```python
from build123d import *

# Parameters (mm, degrees)
F0_W        = 50
F0_H        = 50
F1_DEPTH    = 80
F2_T1_DEPTH = 27.2793198937
F2_T3_DEPTH = 202.8653193294
F2_T5_DEPTH = 172.8653193294
F2_T7_DEPTH = 172.8653193294
F3_SIZE     = 25
F4_SIZE     = 10
F5_SIZE     = 20


# Not quite as in the source:
# - a fillet or chamfer that OpenCascade refuses, or shapes differently, is made with other operations: its cross-section is extruded or revolved along the edge and cut away or added


with BuildPart() as f1:
    # F0 (on Top) → F1 (new body)
    with BuildSketch(Plane.XY):
        Rectangle(F0_W, F0_H)
    extrude(amount=F1_DEPTH)

    # F2: chamfer of 20 x 23.8350718519 on 3 edges, made by hand

    # F2_s2 → F2_t1 (cut)
    with BuildSketch(Plane(origin=(23.3481641649, -33.1608518108, 27.825258524), x_dir=(0.8176584321, 0.5757036463, 0), z_dir=(0.4747146788, -0.6742261621, 0.565742924))):
        Polygon((-13.4400778356, 34.368541497), (17.5629425707, 39.0194717243), (-1.9260049086, 63.2741944877), align=None)
    extrude(amount=F2_T1_DEPTH, mode=Mode.SUBTRACT)

    # F2_s4 → F2_t3 (cut)
    with BuildSketch(Plane.XY.offset(-61.4326596647)):
        Polygon((1.1649281481, -25), (25, -5), (25, -25), align=None)
    extrude(amount=F2_T3_DEPTH, mode=Mode.SUBTRACT)

    # F2_s6 → F2_t5 (cut)
    with BuildSketch(Plane.XZ.offset(-86.4326596647)):
        Polygon((25, 60), (1.1649281481, 80), (25, 80), align=None)
    extrude(amount=F2_T5_DEPTH, mode=Mode.SUBTRACT)

    # F2_s8 → F2_t7 (cut)
    with BuildSketch(Plane.YZ.offset(-86.4326596647)):
        Polygon((-25, 56.1649281481), (-5, 80), (-25, 80), align=None)
    extrude(amount=F2_T7_DEPTH, mode=Mode.SUBTRACT)

    # F3
    f3_edges = [f1.edges().sort_by_distance(p)[0] for p in [
        (-25, 25, 40),
    ]]
    chamfer(f3_edges, length=F3_SIZE)

    # F4
    f4_edges = [f1.edges().sort_by_distance(p)[0] for p in [
        (-12.5, 12.5, 80),
    ]]
    chamfer(f4_edges, length=F4_SIZE)

    # F5
    f5_edges = [f1.edges().sort_by_distance(p)[0] for p in [
        (12.5, 25, 0),
        (-11.917536, -25, 0),
    ]]
    chamfer(f5_edges, length=F5_SIZE)


solid = f1.part
```
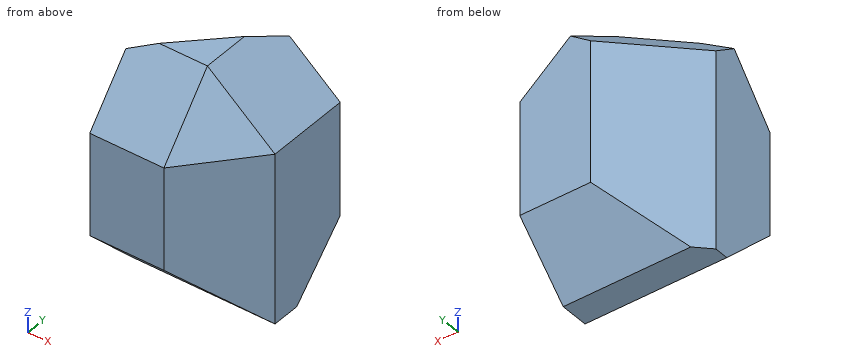
Source: CAD feature listing. Evaluate the final solid. Frame: model axes, mm. Round coordinates to 2 decimals unless told otherwise and drop trailing zeros. Loops run counter-clockwise (first coordinate to the right, second up) from the corner with the lowest first, then second, coordinate; pieces in that order, holes last.
(1) Section query A-A (x = 12.5). Output: boundary loops of the cut face in (y, z).
From the geometry:
outline: (-15.49, 10.49) - (-5, 0) - (5, 0) - (25, 20) - (25, 70.49) - (-5, 70.49) - (-15.49, 57.99) - close
(2) Contact query for flat-ended pins moving along their axis: pin 1 Ø2 at (y, z) = (3.5, 70.5) entering from -X; pin 2 Ø5 at (x, z) = (-18.5, 10) entering from -Y; pin 3 Ø2 at (y, z) = (-18.5, 13.5) entering from +X. Output: stop coordinate, or through.
From the geometry:
pin 1: stops at x = -22.37
pin 2: stops at y = -17.5
pin 3: stops at x = 10.1
(3) Section query D-D (x = 3.5). Output: boundary loops of the cut face in (y, z).
From the geometry:
outline: (-23.04, 18.04) - (-5, 0) - (5, 0) - (25, 20) - (25, 72.47) - (17.13, 78.04) - (-5, 78.04) - (-23.04, 56.54) - close
(4) Section query C-C (y = -17). Output: boundary loops of the cut face in (x, z), and give its area (3 significant figures).
From the geometry:
outline: (-25, 12) - (10.7, 12) - (10.7, 57.7) - (1.16, 65.7) - (-25, 65.7) - close
area: 1,880 mm2
(5) Material intervals for probe 1 along Y at (x, z) = (-5, 20.5); probe 2 along X at (y, z) = (5, 24); probe 3 along X at (y, z) = (15, 30.5), sorted ascending.
From the geometry:
probe 1: y = -25 to 20
probe 2: x = -20 to 25
probe 3: x = -10 to 25
(6) Section query B-B (z = 27.5). Output: boundary loops of the cut face in (x, y), and give its area (3 significant figures).
From the geometry:
outline: (-25, -25) - (1.16, -25) - (25, -5) - (25, 25) - (0, 25) - (-25, 0) - close
area: 1,950 mm2
